Autodesk Inventor part; units mm, degrees
ref_plane "YZ Plane" through (0, 0, 0) normal (1, 0, 0) x (0, 1, 0)
ref_plane "XZ Plane" through (0, 0, 0) normal (0, 1, 0) x (-1, 0, 0)
ref_plane "XY Plane" through (0, 0, 0) normal (0, 0, 1) x (1, 0, 0)
ref_plane "Arbeitsebene1" through (0, 0, 0) normal (0, 0, 1) x (1, 0, 0)
ref_plane "Arbeitsebene2" through (37.9, 18.5, 0) normal (-1, 0, 0) x (0, -1, 0)
sketch "Skizze1" plane through (37.9, 18.5, 0) normal (-1, 0, 0) x (0, -1, 0)
  line L0 (5.15, -4.875) -> (5.15, 0)
  line L1 (13.35, 0) -> (59.85, 0)
  line L2 (13.35, 0) -> (13.35, -4.875)
  arc A0 (5.15, -4.875) -> (13.35, -4.875) centre (9.25, -4.875) ccw
  circle A1 centre (9.25, -4.875) radius 4
  line L3 (5.25, -4.875) -> (13.25, -4.875)
  line L4 (13.25, -4.875) -> (13.25, 1)
  line L5 (13.25, 1) -> (5.25, 1)
  line L6 (5.25, 1) -> (5.25, -4.875)
  line L7 (20.25, 4.5) -> (-1.75, 4.5)
  line L8 (-1.75, 4.5) -> (-1.75, 1)
  line L9 (-1.75, 1) -> (20.25, 1)
  line L10 (20.25, 1) -> (20.25, 4.5)
  line L11 (20.25, 4.5) -> (-1.75, 1) construction
  line L12 (-1.75, 4.5) -> (20.25, 1) construction
  line L13 (20.25, 4.5) -> (21.25, 4.5)
  line L14 (21.25, 4.5) -> (21.25, 1)
  line L15 (21.25, 1) -> (20.25, 1)
  line L16 (20.25, 1) -> (20.25, 4.5)
  line L17 (59.85, -17) -> (-8, -17)
  line L18 (59.85, 0) -> (59.85, -17)
  line L19 (-8, 0) -> (5.15, 0)
  line L20 (-8, -17) -> (-8, 0)
  point P0 (18.5, 0)
  point P1 (0, 0)
  point P2 (59.85, -12)
  point P3 (9.25, 2.75)
  point P4 (13.25, -4.875)
  point P5 (13.25, 1)
  dimension "d0" = 8
  dimension "d1" = 1
  dimension "d2" = 3.5
  dimension "d3" = 11
  dimension "d14" = 1
extrude "Extrusion1" add sketch "Skizze1" against normal blind 9 contours A1 L6 L5 L4 | L5 L9 L8 L7 L10 | L10 L13 L14 L15
sketch "Skizze2" plane through (37.9, -1.75, 4.5) normal (0, 0, 1) x (1, 0, 0)
  circle A0 centre (4.5, 18) radius 1.4
  circle A1 centre (4.5, 4) radius 1.4
  point P0 (-37.9, 1.75)
hole "Bohrung1" at (42.4, 16.25, 4.5) at (42.4, 2.25, 4.5) direction (0, 0, -1) diameter 2.8 depth 8 tip angle 118 counterbore diameter 6.5 counterbore depth 0.5
fillet "Rundung1" radius 1 2 edges at (42.4, 13.25, -4.875) (42.4, 5.25, -4.875)
properties part number "Holisheet_tubeclamp"
Model file for the job. Use its own axes, mm. A direction names the side the tool comes from. Give positions to 0.01 mm unless a question says otherwise; leave off trailing zeros. Write each loop counter-clockwise with the first axis right and the second up, starting at its lowest first coordinate (ties: lowest second). Pieces come first, ordered by that corner, then holes. Notation, with made-up numbers: (68, 50.25) -> (77, 50.25) arc R23 cw to (77, 84.25) -> close; hole circle Ø7 at (1, 65). An arc over 180 degrees is marked (long way). Use CSV: the item, a comma, the result in double quotes. Start each with the question number.
1) Cut at C-C on z = 2.5. List the corners of the cut face in (x, y), plus the area to 3 significant figures.
2) Drill centre lines: L1, parallel to Y at x = 42.4, z = 2; L2, parallel to Y at x = 42.4, z = 4.3; L3, parallel to X at y = 16.25, z = 4.1. Where is each one in solid material? Low to high.
3) Cut at A-A on x = 42.4. List the corners of the cut face in (y, z) (3 decimals).
4) Tool access for faces 1 (the flat face through (41, 18, 1)), 2 (the flat face through (42, 0, 1)), 3 (the cylindrical face through (41.42, -0.85, 4.25)): list every direction of +Z, -Z, +X, -X, +Y, -Y with a clear straight run to the whole face (end or side of a thin tool).
5) Cut at B-B on y = 16.25. List the corners of the cut face in (x, z), plus the area to 4 significant figures.
6) Pin check, flat tips, straight feed: P1, Ø1.5, axis at x = 43.5, z = 0, coming from the -Y side; P2, Ø5, axis at x = 42.4, y = 16.25, coming from the -Z side; P3, Ø1.5, axis at x = 44.5, z = -0.5, coming from the +Y side. Stop position of each tip, or through.
7) Two-plate mould, pull along Y, no slides. Class faces 4 (the cylindrical face through (42.46, 12.68, -1.78)), 5 (the flat face through (42, 13.25, 0)), 6 (the flat face through (42, 9, 4.5)): released by +Y, released by -Y, zero draft, split by the parting line, or undercut.
8) Cut at D-D on z = 4.25. List the corners of the cut face in (x, y), plus the area to 3 significant figures.
Final values:
1,outline,"(37.9, -2.75) -> (46.9, -2.75) -> (46.9, 20.25) -> (37.9, 20.25) -> close; hole circle Ø2.8 at (42.4, 2.25); hole circle Ø2.8 at (42.4, 16.25)"
1,area,"195 mm2"
2,L1,"y = -2.75 to 0.85, 3.65 to 14.85, 17.65 to 20.25"
2,L2,"y = -2.75 to -1, 5.5 to 13, 19.5 to 20.25"
2,L3,"x = 37.9 to 39.15, 45.65 to 46.9"
3,outline,"(-2.75, 1) -> (0.85, 1) -> (0.85, 4) -> (-1, 4) -> (-1, 4.5) -> (-2.75, 4.5) -> close; (3.65, 1) -> (5.25, 1) -> (5.25, -0.881) arc R0.997 ccw to (6.846, -1.678) arc R4 cw to (11.654, -1.678) arc R0.997 ccw to (13.25, -0.881) -> (13.25, 1) -> (14.85, 1) -> (14.85, 4) -> (13, 4) -> (13, 4.5) -> (5.5, 4.5) -> (5.5, 4) -> (3.65, 4) -> close; (17.65, 1) -> (20.25, 1) -> (20.25, 4.5) -> (19.5, 4.5) -> (19.5, 4) -> (17.65, 4) -> close"
4,face 1,"-Z, +X, -X, +Y"
4,face 2,"-Z, +X, -X, -Y"
4,face 3,"+Z"
5,outline,"(37.9, 1) -> (41, 1) -> (41, 4) -> (39.15, 4) -> (39.15, 4.5) -> (37.9, 4.5) -> close; (43.8, 1) -> (46.9, 1) -> (46.9, 4.5) -> (45.65, 4.5) -> (45.65, 4) -> (43.8, 4) -> close"
5,area,"19.85 mm2"
6,P1,"stops at y = 5.25"
6,P2,"stops at z = 1"
6,P3,"stops at y = 13.25"
7,face 4,"undercut"
7,face 5,"released by +Y"
7,face 6,"zero draft"
8,outline,"(37.9, -2.75) -> (46.9, -2.75) -> (46.9, 20.25) -> (37.9, 20.25) -> close; hole circle Ø6.5 at (42.4, 2.25); hole circle Ø6.5 at (42.4, 16.25)"
8,area,"141 mm2"
